Build history of the part. All positions in model axes, mm. Face numbers are marked on the shaded views. A direction names the side the tool comes from. Coordinates: 2 decimals unless noted, no trailing zeros. Loops run counter-clockwise (first coordinate to the right, second up) from the corner with the lowest first, then second, coordinate; pieces in that order, holes last. Notation, with made-up numbers: (19.5, -15) -> (68.5, -15) arc R17 ccw to (68.5, 6) -> close; hole circle Ø9 at (30, -17). An arc over 180 degrees is marked (long way). One line per item, written item: value. Start each with the question number.
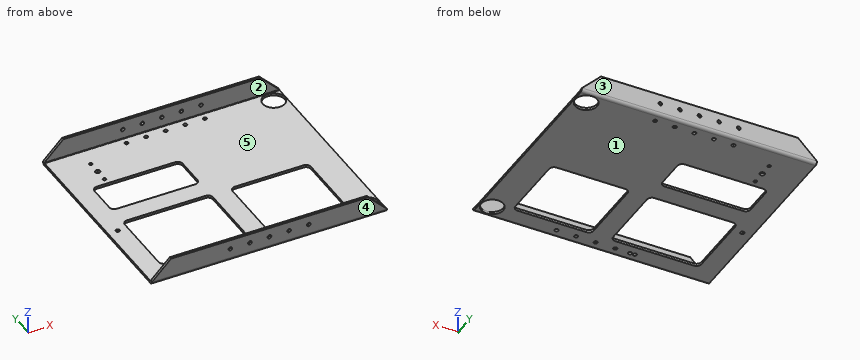
```python
from build123d import *

# Parameters (mm, degrees)
SKETCH1_W                    = 304.8
SKETCH1_H                    = 266.7
SKETCH1_R                    = 14.2875
SKETCH1_R_2                  = 3.175
SKETCH1_R_3                  = 2.0955
SKETCH1_R_4                  = 2.3876
SKETCH1_R_5                  = 2.5527
BASE_FLANGE1_DEPTH           = 3.175
EDGE_FLANGE1_STRIP_W         = 14.1732
EDGE_FLANGE1_STRIP_H         = 3.175
EDGE_FLANGE1_STRIP_CUT_DEPTH = 304.8
EDGE_FLANGE1_DEPTH           = 304.8
EDGE_FLANGE2_STRIP_W         = 14.1732
EDGE_FLANGE2_STRIP_H         = 3.175
EDGE_FLANGE2_STRIP_CUT_DEPTH = 304.8
EDGE_FLANGE2_DEPTH           = 304.8
CUT_EXTRUDE1_DEPTH           = 406.80425084
CUT_EXTRUDE2_DEPTH           = 406.80425084
SKETCH15_R                   = 2.3876
CUT_EXTRUDE3_DEPTH           = 406.80425084


# Sheet-metal steps are written as plain solids
with BuildPart() as part:
    # Sketch1 → Base-Flange1 (new body)
    with BuildSketch(Plane.XY):
        with Locations((152.4, 133.35)):
            Rectangle(SKETCH1_W, SKETCH1_H)
        with Locations((289.56, 18.415)):
            Circle(SKETCH1_R, mode=Mode.SUBTRACT)
        with Locations(Location((289.56, 248.285, 0), (0, 0, 180))):
            Circle(SKETCH1_R, mode=Mode.SUBTRACT)
        with Locations((46.355, 220.345)):
            Circle(SKETCH1_R_2, mode=Mode.SUBTRACT)
        with Locations((46.355, 237.187832598)):
            Circle(SKETCH1_R_3, mode=Mode.SUBTRACT)
        with Locations((46.355, 203.502167402)):
            Circle(SKETCH1_R_3, mode=Mode.SUBTRACT)
        with Locations((152.4, 12.7)):
            Circle(SKETCH1_R_4, mode=Mode.SUBTRACT)
        with Locations((177.8, 12.7)):
            Circle(SKETCH1_R_4, mode=Mode.SUBTRACT)
        with Locations((203.2, 12.7)):
            Circle(SKETCH1_R_4, mode=Mode.SUBTRACT)
        with Locations((127, 12.7)):
            Circle(SKETCH1_R_4, mode=Mode.SUBTRACT)
        with Locations((101.6, 12.7)):
            Circle(SKETCH1_R_4, mode=Mode.SUBTRACT)
        with Locations(Location((101.6, 254, 0), (0, 0, 180))):
            Circle(SKETCH1_R_4, mode=Mode.SUBTRACT)
        with Locations(Location((127, 254, 0), (0, 0, 180))):
            Circle(SKETCH1_R_4, mode=Mode.SUBTRACT)
        with Locations(Location((203.2, 254, 0), (0, 0, 180))):
            Circle(SKETCH1_R_4, mode=Mode.SUBTRACT)
        with Locations(Location((177.8, 254, 0), (0, 0, 180))):
            Circle(SKETCH1_R_4, mode=Mode.SUBTRACT)
        with Locations(Location((152.4, 254, 0), (0, 0, 180))):
            Circle(SKETCH1_R_4, mode=Mode.SUBTRACT)
        with Locations((107.95, 12.7)):
            Circle(SKETCH1_R_5, mode=Mode.SUBTRACT)
        with Locations((12.7, 107.95)):
            Circle(SKETCH1_R_5, mode=Mode.SUBTRACT)
        with BuildLine():
            Line((171.45, 120.65), (260.35, 120.65))
            ThreePointArc((260.35, 120.65), (264.840128061, 118.790128061), (266.7, 114.3))
            Line((266.7, 114.3), (266.7, 31.75))
            ThreePointArc((266.7, 31.75), (264.840128061, 27.259871939), (260.35, 25.4))
            Line((260.35, 25.4), (171.45, 25.4))
            ThreePointArc((171.45, 25.4), (166.959871939, 27.259871939), (165.1, 31.75))
            Line((165.1, 31.75), (165.1, 114.3))
            ThreePointArc((165.1, 114.3), (166.959871939, 118.790128061), (171.45, 120.65))
        make_face(mode=Mode.SUBTRACT)
        with BuildLine():
            Line((31.75, 120.65), (133.35, 120.65))
            ThreePointArc((133.35, 120.65), (137.840128061, 118.790128061), (139.7, 114.3))
            Line((139.7, 114.3), (139.7, 31.75))
            ThreePointArc((139.7, 31.75), (137.840128061, 27.259871939), (133.35, 25.4))
            Line((133.35, 25.4), (31.75, 25.4))
            ThreePointArc((31.75, 25.4), (27.259871939, 27.259871939), (25.4, 31.75))
            Line((25.4, 31.75), (25.4, 114.3))
            ThreePointArc((25.4, 114.3), (27.259871939, 118.790128061), (31.75, 120.65))
        make_face(mode=Mode.SUBTRACT)
        with BuildLine():
            Line((31.75, 194.945), (133.35, 194.945))
            ThreePointArc((133.35, 194.945), (137.840128061, 193.085128061), (139.7, 188.595))
            Line((139.7, 188.595), (139.7, 152.4))
            ThreePointArc((139.7, 152.4), (137.840128061, 147.909871939), (133.35, 146.05))
            Line((133.35, 146.05), (31.75, 146.05))
            ThreePointArc((31.75, 146.05), (27.259871939, 147.909871939), (25.4, 152.4))
            Line((25.4, 152.4), (25.4, 188.595))
            ThreePointArc((25.4, 188.595), (27.259871939, 193.085128061), (31.75, 194.945))
        make_face(mode=Mode.SUBTRACT)
    extrude(amount=-BASE_FLANGE1_DEPTH)

    # Edge-Flange1 strip (across the edge) → Edge-Flange1 strip cut (cut)
    with BuildSketch(Plane(origin=(304.8, 266.7, 0), x_dir=(0, -1, 0), z_dir=(-1, 0, 0))):
        with Locations((-3.175, -1.5875)):
            Rectangle(EDGE_FLANGE1_STRIP_W, EDGE_FLANGE1_STRIP_H)
    extrude(amount=EDGE_FLANGE1_STRIP_CUT_DEPTH, mode=Mode.SUBTRACT)

    # Edge-Flange1 section (across the edge) → Edge-Flange1 (add)
    with BuildSketch(Plane(origin=(304.8, 266.7, 0), x_dir=(0, -1, 0), z_dir=(-1, 0, 0))):
        with BuildLine():
            Line((0, 0.7366), (0, 25.4))
            Line((0, 25.4), (3.175, 25.4))
            Line((3.175, 25.4), (3.175, 0.7366))
            ThreePointArc((3.175, 0.7366), (3.390745145, 0.215745145), (3.9116, 0))
            Line((3.9116, 0), (3.9116, -3.175))
            ThreePointArc((3.9116, -3.175), (1.145681115, -2.029318885), (0, 0.7366))
        make_face()
    extrude(amount=EDGE_FLANGE1_DEPTH)

    # Edge-Flange2 strip (across the edge) → Edge-Flange2 strip cut (cut)
    with BuildSketch(Plane.YZ):
        with Locations((-3.175, -1.5875)):
            Rectangle(EDGE_FLANGE2_STRIP_W, EDGE_FLANGE2_STRIP_H)
    extrude(amount=EDGE_FLANGE2_STRIP_CUT_DEPTH, mode=Mode.SUBTRACT)

    # Edge-Flange2 section (across the edge) → Edge-Flange2 (add)
    with BuildSketch(Plane.YZ):
        with BuildLine():
            Line((0, 0.7366), (0, 25.4))
            Line((0, 25.4), (3.175, 25.4))
            Line((3.175, 25.4), (3.175, 0.7366))
            ThreePointArc((3.175, 0.7366), (3.390745145, 0.215745145), (3.9116, 0))
            Line((3.9116, 0), (3.9116, -3.175))
            ThreePointArc((3.9116, -3.175), (1.145681115, -2.029318885), (0, 0.7366))
        make_face()
    extrude(amount=EDGE_FLANGE2_DEPTH)

    # Sketch12 → Cut-Extrude1 (cut, through all)
    with BuildSketch(Plane(origin=(0, 0, 0), x_dir=(-1, 0, 0), z_dir=(0, -1, 0))):
        Polygon((-304.8, -0.7366), (-280.1366, -25.4), (-304.8, -25.4), align=None)
    extrude(amount=-CUT_EXTRUDE1_DEPTH, mode=Mode.SUBTRACT)

    # Sketch14 → Cut-Extrude2 (cut, through all)
    with BuildSketch(Plane.XZ):
        Polygon((0, 0.7366), (24.6634, 25.4), (0, 25.4), align=None)
    extrude(amount=-CUT_EXTRUDE2_DEPTH, mode=Mode.SUBTRACT)

    # Sketch15 → Cut-Extrude3 (cut, through all)
    with BuildSketch(Plane.XZ):
        with Locations(Location((152.4, 13.0683, 0), (0, 0, 270))):
            Circle(SKETCH15_R)
        with Locations(Location((177.8, 13.0683, 0), (0, 0, 270))):
            Circle(SKETCH15_R)
        with Locations(Location((203.2, 13.0683, 0), (0, 0, 270))):
            Circle(SKETCH15_R)
        with Locations(Location((127, 13.0683, 0), (0, 0, 270))):
            Circle(SKETCH15_R)
        with Locations(Location((101.6, 13.0683, 0), (0, 0, 270))):
            Circle(SKETCH15_R)
    extrude(amount=-CUT_EXTRUDE3_DEPTH, mode=Mode.SUBTRACT)


solid = part.part
```
Item 1: Two-plate mould, pull along Y, no slides. Class the marked faces 1, 2 and 3: +Y half, -Y half, draft (parallel to the pull), parting line (faces both ways), or undercut.
Item 2: Band-saw the part on B-B, the plane x = 289.56. Count the separate pieces of the cut face and the enclosed holes in it, and give its area (3 significant figures).
Item 3: Tool access for the marked faces 4 and 5: list every direction of +Z, -Z, +X, -X, +Y, -Y with a clear straight run to the whole face (end or side of a thin tool).
Item 4: Probe probe 1 along X at (y, z) = (85.5, -2); probe 2 along Y at (x, z) = (172, 16.25) (3 decimals); probe 3 along Y at (x, z) = (152.4, -1.85). List the from-to ranges inside material, lowest first.
Item 5: Drop flat-ended pins along their axis: pin 1 Ø4 at (x, z) = (177.8, 13.07) entering from +Y; pin 2 Ø10 at (x, y) = (106.5, 139.5) entering from +Z; pin 3 Ø1 at (x, z) = (66, -2.5) entering from +Y; pin 4 Ø3.5 at (x, z) = (63, -1.5) entering from -Y. Give the stop position or say it passes through.
Item 6: Band-saw the part on A-A, the plane y = 101. List the corners of the cut face in (x, z) (3 decimals).
Worked out:
1. face 1: draft
1. face 2: undercut
1. face 3: +Y half
2. separate pieces: 3
2. enclosed holes: 0
2. area: 760 mm²
3. face 4: +Z, -Z, +X, -X, -Y
3. face 5: +Z, +X, -X
4. probe 1: x = 0 to 25.4, 139.7 to 165.1, 266.7 to 304.8
4. probe 2: y = 0 to 3.175, 263.525 to 266.7
4. probe 3: y = 0.98 to 10.31, 15.09 to 251.61, 256.39 to 265.72
5. pin 1: passes through
5. pin 2: stops at z = 0
5. pin 3: stops at y = 265.58
5. pin 4: stops at y = 0.03
6. outline: (0, -3.175) -> (25.4, -3.175) -> (25.4, 0) -> (0, 0) -> close; (139.7, -3.175) -> (165.1, -3.175) -> (165.1, 0) -> (139.7, 0) -> close; (266.7, -3.175) -> (304.8, -3.175) -> (304.8, 0) -> (266.7, 0) -> close
